from build123d import *

# Parameters (mm, degrees)
F0_W     = 900
F0_H     = 200
F1_DEPTH = 250
F3_DEPTH = 100
F4_R     = 10


with BuildPart() as f1:
    # F0 (on Front) → F1 (new body, symmetric)
    with BuildSketch(Plane.XZ):
        Rectangle(F0_W, F0_H)
    extrude(amount=F1_DEPTH, both=True)

    # F2 (on face) → F3 (cut)
    with BuildSketch(Plane.XY.offset(100)):
        Polygon((-350, -150), (350, -150), (350, 50), (250, 150), (0, 150), (-250, 150), (-350, 50), align=None)
    extrude(amount=-F3_DEPTH, mode=Mode.SUBTRACT)

    # F4
    f4_edges = [f1.edges().sort_by_distance(p)[0] for p in [
        (450, -250, 0),
        (-450, -250, 0),
        (450, 250, 0),
        (-450, 250, 0),
    ]]
    fillet(f4_edges, radius=F4_R)


solid = f1.part
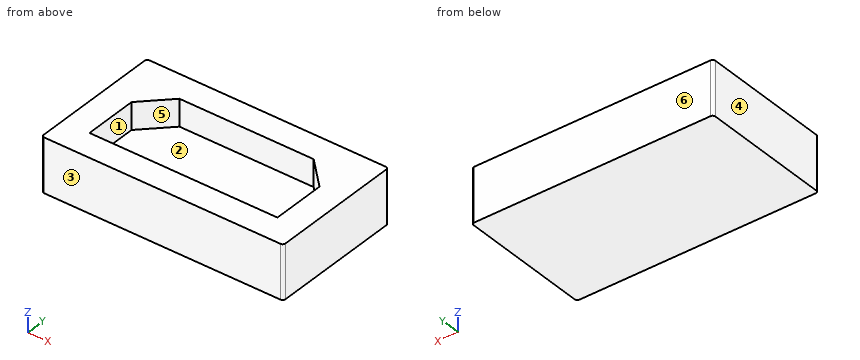
Verification items for the finished model (mm, model axes). Face numbers are marked on the shaded views. A direction names the side the tool comes from. Coordinates: 2 decimals unless noted, no trailing zeros. Order: outer loops, then holes, each group sorted by start corner. A loop starts at its lowest first (then second) coordinate and runs counter-clockwise, first axis right, second up.
1. Set-up check for the marked faces 5 and 6: record each of +Z, -Z, +X, -X, +Y, -Y from which the full face is reachable in a straight line by a thin tool's end or side.
Results found:
face 5: +Z
face 6: +Z, -Z, +X, -X, +Y
2. Release check for a two-part mould opening along Y. For the marked faces 1, 2, 3 and 4 record: +Y half, -Y half, draft (parallel to the pull), parting line (faces both ways), or undercut.
Results found:
face 1: undercut
face 2: undercut
face 3: -Y half
face 4: draft
3. Sectioned sample at A-A, the plane y = -104. Record the cut outline in (x, z), and give its area (3 significant figures).
Results found:
outline: (-450, -100) - (450, -100) - (450, 100) - (350, 100) - (350, 0) - (-350, 0) - (-350, 100) - (-450, 100) - close
area: 110,000 mm2
4. Go/stop test with a flat-tipped pin: pin 1 Ø5 at (x, y) = (-142, -120.5) entering from +Z. Record where the tip stops, or that it passes through.
Results found:
pin 1: stops at z = 0
5. Sectioned sample at B-B, the plane z = 33. Record the cut outline in (x, y), and give its area (3 significant figures).
Results found:
outline: (-450, -240) arc R10 ccw to (-440, -250) - (440, -250) arc R10 ccw to (450, -240) - (450, 240) arc R10 ccw to (440, 250) - (-440, 250) arc R10 ccw to (-450, 240) - close; hole (-350, -150) - (350, -150) - (350, 50) - (250, 150) - (-250, 150) - (-350, 50) - close
area: 250,000 mm2
6. Sectioned sample at C-C, the plane x = 21.5. Record the cut outline in (y, z).
Results found:
outline: (-250, -100) - (250, -100) - (250, 100) - (150, 100) - (150, 0) - (-150, 0) - (-150, 100) - (-250, 100) - close
7. Scan lines: line 1 (Y direction, x = 191, z = 42.5); line 2 (X direction, y = -86, z = 49); line 3 (Z direction, x = 254, y = 124). Record each from-to range of solid material in increasing order.
Results found:
line 1: y = -250 to -150, 150 to 250
line 2: x = -450 to -350, 350 to 450
line 3: z = -100 to 0
